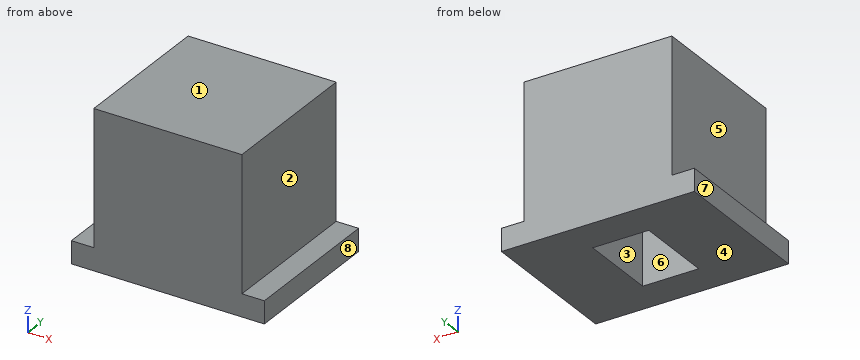
from build123d import *

# Parameters (mm, degrees)
SKETCH014_W      = 2.5
SKETCH014_H      = 3.5
EXTRUDE015_DEPTH = 4.5
EXTRUDE014_DEPTH = 6.6


with BuildPart() as extrude015:
    # Sketch014 → Extrude015 (new body)
    with BuildSketch(Plane(origin=(0, 0, -10), x_dir=(1, 0, 0), z_dir=(0, 0, -1))):
        Rectangle(SKETCH014_W, SKETCH014_H)
    extrude(amount=-EXTRUDE015_DEPTH)


with BuildPart() as extrude015_1:
    # Extrude015 placement: moved
    add(extrude015.part.moved(Location((0, 0, 10))))


with BuildPart() as cut023:
    # Sketch013 → Extrude014 (new body)
    with BuildSketch(Plane.XZ.offset(10)):
        Polygon((-3.3, 7), (3.3, 7), (3.3, 1), (4.3, 1), (4.3, 0), (-4.3, 0), (-4.3, 1), (-3.3, 1), align=None)
    extrude(amount=-EXTRUDE014_DEPTH)


with BuildPart() as cut023_1:
    # Extrude014 placement: moved
    add(cut023.part.moved(Location((0, 6.75, 0))))

    # Cut023: cut Extrude015
    add(extrude015_1.part, mode=Mode.SUBTRACT)


solid = cut023_1.part
Source: CAD feature listing. Evaluate the final solid. Frame: model axes, mm. Face numbers are marked on the shaded views. A direction names the side the tool comes from. Give positions to 0.01 mm unless a question says otherwise; leave off trailing zeros. Write each loop counter-clockwise with the first axis right and the second up, starting at its lowest first coordinate (ties: lowest second). Pieces come first, ordered by that corner, then holes. Notation, with made-up numbers: M 89.25,-8.75 L 101.25,-8.75 A15 ccw 101.25,1.25 Z; hole C 12,25.5 d9. An arc over 180 degrees is marked long. Return JSON: item names as keys, results as strings. Group by question number.
1) Cut plane C-C, the plane y = 0.25. Output: boundary loops of the cut face in (x, z), then the cut area to 4 significant figures.
2) Cut plane B-B, the plane x = 0. Output: boundary loops of the cut face in (y, z).
3) Set-up query: the marked faces 1, 2, 3, 4 and 5. Return all of +Z, -Z, +X, -X, +Y, -Y with unobstructed straight access to the full face (end or side cutting, diameter ignored); none if empty.
4) First-contact query: pin 1 Ø1.8 at (y, z) = (1.5, 4) entering from +X; pin 2 Ø1.1 at (x, y) = (4, -0.5) entering from +Z; pin 3 Ø1.2 at (x, y) = (-0.5, -0.5) entering from -Z. Flat tips, straight axial feed; report the tip coordinate or a pass-through.
5) Cut plane D-D, the plane z = 5.25. Output: boundary loops of the cut face in (x, y).
6) Ray query, L1, parallel to Y at x = 0.75, z = 1.5; L2, parallel to X at y = -1.25, z = 3.5; L3, parallel to X at y = 2.25, z = 4.75. Return the intervals inside material, ascending.
7) Cut plane A-A, the plane z = 2. Output: boundary loops of the cut face in (x, y), then the cut area to 3 significant figures.
8) Draft query along X for the marked faces 6, 7 and 8. Return one class per face: released by +X, released by -X, zero draft, split by the parting line, or undercut.
Data:
{
 "1": {"outline": "M -4.3,0 L -1.25,0 L -1.25,4.5 L 1.25,4.5 L 1.25,0 L 4.3,0 L 4.3,1 L 3.3,1 L 3.3,7 L -3.3,7 L -3.3,1 L -4.3,1 Z", "area": "36.95 mm²"},
 "2": {"outline": "M -3.25,0 L -1.75,0 L -1.75,4.5 L 1.75,4.5 L 1.75,0 L 3.35,0 L 3.35,7 L -3.25,7 Z"},
 "3": {"face 1": "+Z, +X, -X, +Y, -Y", "face 2": "+Z, +X, +Y, -Y", "face 3": "-Z", "face 4": "-Z, +X, -X, +Y, -Y", "face 5": "+Z, -X, +Y, -Y"},
 "4": {"pin 1": "stops at x = 3.3", "pin 2": "stops at z = 1", "pin 3": "stops at z = 4.5"},
 "5": {"outline": "M -3.3,-3.25 L 3.3,-3.25 L 3.3,3.35 L -3.3,3.35 Z"},
 "6": {"L1": "y = -3.25 to -1.75, 1.75 to 3.35", "L2": "x = -3.3 to -1.25, 1.25 to 3.3", "L3": "x = -3.3 to 3.3"},
 "7": {"outline": "M -3.3,-3.25 L 3.3,-3.25 L 3.3,3.35 L -3.3,3.35 Z; hole M -1.25,-1.75 L 1.25,-1.75 L 1.25,1.75 L -1.25,1.75 Z", "area": "34.8 mm²"},
 "8": {"face 6": "undercut", "face 7": "released by -X", "face 8": "released by +X"}
}
